Autodesk Inventor part; units mm, degrees
ref_plane "YZ Plane" through (0, 0, 0) normal (1, 0, 0) x (0, 1, 0)
ref_plane "XZ Plane" through (0, 0, 0) normal (0, 1, 0) x (-1, 0, 0)
ref_plane "XY Plane" through (0, 0, 0) normal (0, 0, 1) x (1, 0, 0)
sketch "草圖1" plane through (0, 0, 0) normal (0, 1, 0) x (-1, 0, 0)
  circle A0 centre (0, 0) radius 20
  line L0 (0, -20) -> (30, -20)
  line L1 (30, -20) -> (30, 20)
  line L2 (30, 20) -> (0, 20)
  line L3 (0, 20) -> (0, -20)
  point P0 (0, 20)
  dimension "d0" = 40
  dimension "d1" = 30
extrude "擠出1" add sketch "草圖1" along normal blind 30
sketch "草圖2" plane through (-30, 0, 20) normal (0, 0, 1) x (1, 0, 0)
  line L0 (0, 0) -> (0, 30)
  line L1 (0, 30) -> (30, 30)
  line L2 (30, 0) -> (30, 30)
  line L3 (30, 0) -> (0, 0)
  line L4 (10, 37.5679) -> (66.1175, 37.5679)
  line L5 (66.1175, 37.5679) -> (66.1175, 10)
  line L6 (66.1175, 10) -> (10, 10)
  line L7 (10, 10) -> (10, 37.5679)
  dimension "d4" = 10
  dimension "d5" = 10
extrude "擠出2" cut sketch "草圖2" against normal blind 48.25 contours L7 L4 L5 L6 L2 L1 | L1 L2 L6 L7
sketch "草圖3" plane through (-20, 10, 20) normal (1, 0, 0) x (0, 0, -1)
  line L0 (0, 0) -> (40, 0)
  line L1 (40, 20) -> (40, 0)
  line L2 (0, 20) -> (40, 20)
  line L3 (0, 0) -> (0, 20)
  line L4 (0, -10) -> (0, 0)
  line L5 (40, -10) -> (0, -10)
  line L6 (40, 0) -> (40, -10)
  line L7 (40, 20) -> (0, 20)
  line L8 (0, 20) -> (10, 20)
  line L9 (10, 20) -> (10, 10)
  line L10 (10, 10) -> (0, 10)
  line L11 (0, 10) -> (0, 20)
  point P0 (20, -10)
  dimension "d8" = 10
  dimension "d9" = 10
extrude "擠出3" cut sketch "草圖3" against normal blind 10 contours L3 L2 L9 L10
sketch "草圖4" plane through (-20, 10, 20) normal (0, 1, 0) x (1, 0, 0)
  arc A0 (20, 0) -> (20, 40) centre (20, 20) ccw
hole "孔1" at (0, 10, 0) direction (0, -1, 0) diameter 20 end through all
properties part number "35" material "鋼、碳鋼"
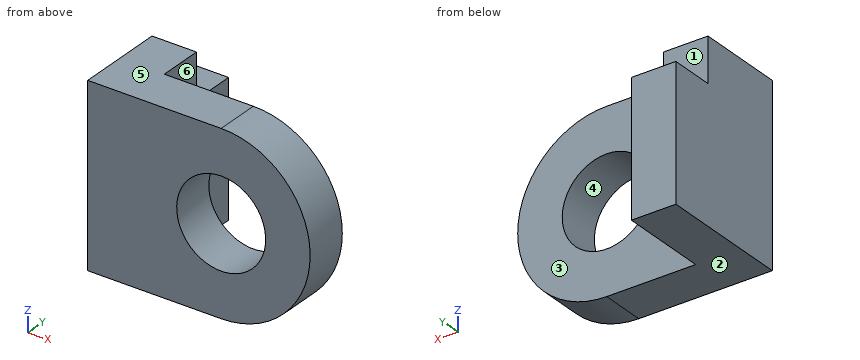
Part model, mm, in its own coordinate system. Face numbers are marked on the shaded views. A direction names the side the tool comes from. Round coordinates to 2 decimals unless told otherwise and drop trailing zeros. Write each loop counter-clockwise with the first axis right and the second up, starting at its lowest first coordinate (ties: lowest second). Pieces come first, ordered by that corner, then holes. Notation, with made-up numbers: (8.5, 31) -> (13.5, 31) arc R19 cw to (13.5, 42) -> close; hole circle Ø1 at (5.5, -38). An arc over 180 degrees is marked (long way). Return JSON: item names as keys, results as strings. Group by question number.
Q1. Which spindle directions (+Z, -Z, +X, -X, +Y, -Y) get a long thin tool onto all of the face, cutting with end or side? Do the marked faces 1, 2 and 3. Say none if no direction does.
Q2. Pin check, flat tips, straight feed: pin 1 (3 mm diameter, centred on x = -25, z = 14.5, fed in from +Y); pin 2 (23 mm diameter, centred on x = 0, z = 0, fed in from +Y); pin 3 (1 mm diameter, centred on y = 7, z = 3, fed in from +X). Stop position of each tip, or through.
Q3. Saw through at D-D on x = -23. Write the cut outline in (y, z).
Q4. Saw through at B-B on x = 5. Write the cut outline in (y, z).
Q5. Saw through at A-A on z = 0. Write the cut outline in (x, y), plus the area to 3 significant figures.
Q6. Saw through at C-C on y = 5. Write the cut outline in (x, z), plus the area to 3 significant figures.
Q7. Probe L1, parallel to Z at x = 0, y = 6; L2, parallel to X at y = 3.5, z = 0; L3, parallel to Y at x = -12.5, z = 3.5. List the from-to ranges inside material, lowest first. Write a range as [from, to].
Q8. Mould opens along Z. For the marked faces 4, 5 and 6 say: pulls with the +Z half, pulls with the -Z half, needs draft (parallel to the pull), parting line crosses it, or undercut.
Answer:
{
 "1": {"face 1": "+Z, +X, -X, +Y", "face 2": "-Z, +X, -X, +Y, -Y", "face 3": "+Z, -Z, +X, +Y"},
 "2": {"pin 1": "y = 20", "pin 2": "y = 10", "pin 3": "x = 19.84"},
 "3": {"outline": "(0, -20) -> (30, -20) -> (30, 10) -> (20, 10) -> (20, 20) -> (0, 20) -> close"},
 "4": {"outline": "(0, -19.36) -> (10, -19.36) -> (10, -8.66) -> (0, -8.66) -> close; (0, 8.66) -> (10, 8.66) -> (10, 19.36) -> (0, 19.36) -> close"},
 "5": {"outline": "(-30, 0) -> (-10, 0) -> (-10, 10) -> (-20, 10) -> (-20, 30) -> (-30, 30) -> close; (10, 0) -> (20, 0) -> (20, 10) -> (10, 10) -> close", "area": "500 mm2"},
 "6": {"outline": "(-30, -20) -> (0, -20) arc R20 ccw to (0, 20) -> (-30, 20) -> close; hole circle Ø20 at (0, 0)", "area": "1,510 mm2"},
 "7": {"L1": "[-20, -10], [10, 20]", "L2": "[-30, -10], [10, 20]", "L3": "[0, 10]"},
 "8": {"face 4": "undercut", "face 5": "pulls with the +Z half", "face 6": "needs draft"}
}
